Answer from the drawing. Dimensions are ordinates in mm from the lowest x, y and z of the part. A direction names the side the tool comes from. Coordinates: 2 decimals unless noted, no trailing zeros. Loops run counter-clockwise (first coordinate to the right, second up) from the corner with the lowest first, then second, coordinate; pieces in that order, holes last. Notation, with made-up numbers: (52, -33.75) -> (95, -33.75) arc R12 ccw to (95, -15.75) -> close; hole circle Ø8 at (-15, 72). An arc over 180 degrees is marked (long way). Use a Markdown table: item, result.
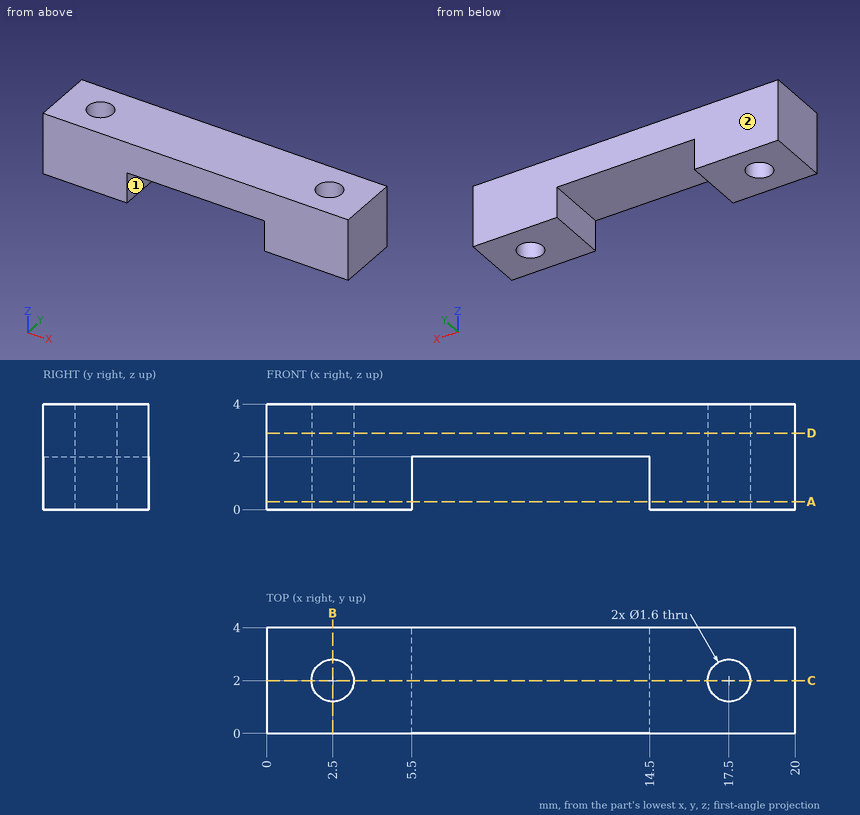
Q1. Section C-C on y = 2 is taken. Determine the outline of the cut face in (x, z), and give its area (3 significant figures).
Solved:
| item | result |
|---|---|
| outline | (0, 0) -> (1.7, 0) -> (1.7, 4) -> (0, 4) -> close; (3.3, 0) -> (5.5, 0) -> (5.5, 2) -> (14.5, 2) -> (14.5, 0) -> (16.7, 0) -> (16.7, 4) -> (3.3, 4) -> close; (18.3, 0) -> (20, 0) -> (20, 4) -> (18.3, 4) -> close |
| area | 49.2 mm² |
Q2. Section A-A on z = 0.3 is taken. Determine the outline of the cut face in (x, y), and give its area (3 significant figures).
Solved:
| item | result |
|---|---|
| outline | (0, 0) -> (5.5, 0) -> (5.5, 4) -> (0, 4) -> close; (14.5, 0) -> (20, 0) -> (20, 4) -> (14.5, 4) -> close; hole circle Ø1.6 at (2.5, 2); hole circle Ø1.6 at (17.5, 2) |
| area | 40.0 mm² |
Q3. Given pin 1 Ø1.8 at (x, y) = (2.5, 2) entering from +Z, flat-ended and moving along its own axis, determine where the tip first touches the part or whether it passes through.
Solved:
| item | result |
|---|---|
| pin 1 | z = 4 |
Q4. Consider line 1 (X direction, y = 2, z = 2.35); line 2 (X direction, y = 2, z = 1.2); line 3 (X direction, y = 1.1, z = 0.9). Determine where each line is inside the solid, lowest interval first. Write a range as [from, to].
Solved:
| item | result |
|---|---|
| line 1 | [0, 1.7], [3.3, 16.7], [18.3, 20] |
| line 2 | [0, 1.7], [3.3, 5.5], [14.5, 16.7], [18.3, 20] |
| line 3 | [0, 5.5], [14.5, 20] |
Q5. Section D-D on z = 2.9 is taken. Determine the outline of the cut face in (x, y), and give its area (3 significant figures).
Solved:
| item | result |
|---|---|
| outline | (0, 0) -> (20, 0) -> (20, 4) -> (0, 4) -> close; hole circle Ø1.6 at (2.5, 2); hole circle Ø1.6 at (17.5, 2) |
| area | 76.0 mm² |
Q6. For the marked faces 1 and 2, determine the directions among +Z, -Z, +X, -X, +Y, -Y from which every point of the face is accessible in a straight line to the end or side of a thin tool.
Solved:
| item | result |
|---|---|
| face 1 | -Z, +Y, -Y |
| face 2 | +Z, -Z, +X, -X, +Y |
Q7. Section B-B on x = 2.5 is taken. Determine the outline of the cut face in (y, z).
Solved:
| item | result |
|---|---|
| outline | (0, 0) -> (1.2, 0) -> (1.2, 4) -> (0, 4) -> close; (2.8, 0) -> (4, 0) -> (4, 4) -> (2.8, 4) -> close |
